Read the model definition and answer for the solid it produces. Units are mm, in the model's axes. Face numbers are marked on the shaded views. A direction names the side the tool comes from. Coordinates: 2 decimals unless noted, no trailing zeros. Loops run counter-clockwise (first coordinate to the right, second up) from the corner with the lowest first, then second, coordinate; pieces in that order, holes last.
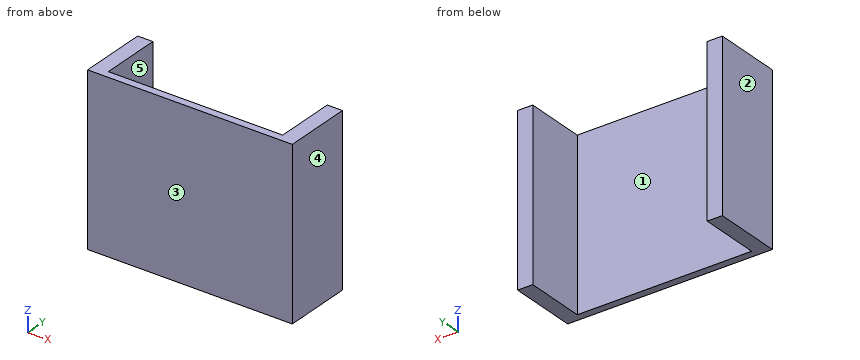
Autodesk Inventor part; units mm, degrees
ref_plane "YZ Plane" through (0, 0, 0) normal (1, 0, 0) x (0, 1, 0)
ref_plane "XZ Plane" through (0, 0, 0) normal (0, 1, 0) x (-1, 0, 0)
ref_plane "XY Plane" through (0, 0, 0) normal (0, 0, 1) x (1, 0, 0)
sketch "Sketch1" plane through (0, 0, 0) normal (0, 1, 0) x (-1, 0, 0)
  line L0 (86.4286, 125.7143) -> (-143.5714, 125.7143)
  line L1 (-143.5714, 125.7143) -> (-143.5714, -94.2857)
  line L2 (-143.5714, -94.2857) -> (86.4286, -94.2857)
  line L3 (86.4286, -94.2857) -> (86.4286, 125.7143)
  point P0 (0, 0)
  dimension "d0" = 220
  dimension "d1" = 230
extrude "Extrusion1" add sketch "Sketch1" along normal blind 10
sketch "Sketch5" plane through (-86.4286, 0, 125.7143) normal (0, 0, 1) x (1, 0, 0)
  line L0 (0, 0) -> (0, 10)
  line L1 (0, 0) -> (-20, 0)
  line L2 (-20, 0) -> (-20, 90)
  line L3 (-20, 90) -> (0, 90)
  line L4 (0, 90) -> (0, 0)
  line L5 (230, 0) -> (0, 0)
  line L6 (230, 0) -> (250, 0)
  line L7 (250, 0) -> (250, 90)
  line L8 (250, 90) -> (230, 90)
  line L9 (230, 90) -> (230, 0)
  point P0 (86.4286, 0)
  dimension "d22" = 90
  dimension "d23" = 20
  dimension "d24" = 20
extrude "Extrusion5" add sketch "Sketch5" against normal up to surface (220 mm away)
properties part number "Podkladka" material "Aluminum 6061"
Item 1: A cutting plane is placed at A-A on y = 23.5. Determine the outline of the cut face in (x, z).
Numbers:
outline: (-106.43, -94.29) - (-86.43, -94.29) - (-86.43, 125.71) - (-106.43, 125.71) - close; (143.57, -94.29) - (163.57, -94.29) - (163.57, 125.71) - (143.57, 125.71) - close
Item 2: A cutting plane is placed at B-B on z = 2.5. Determine the outline of the cut face in (x, y), then the cut area to 3 significant figures.
Numbers:
outline: (-106.43, 0) - (163.57, 0) - (163.57, 90) - (143.57, 90) - (143.57, 10) - (-86.43, 10) - (-86.43, 90) - (-106.43, 90) - close
area: 5,900 mm2
Item 3: Which of the six approach directions +Z, -Z, +X, -X, +Y, -Y give full straight-line access (tool end or side, diameter ignored) to the marked faces 1 and 2?
Numbers:
face 1: +Z, -Z, +Y
face 2: +Z, -Z, -X, +Y, -Y
Item 4: Given pin 1 (12 mm diameter, centred on x = 19.5, z = -72.5, fed in from +Y), flat-ended and moving along its own axis, determine where the tip first touches the part or whether it passes through.
Numbers:
pin 1: stops at y = 10
Item 5: Find the intervals of material crossed by line 1 along X through (y, z) = (82, -8); line 2 along Y through (x, z) = (57.5, 47), in increasing order.
Numbers:
line 1: x = -106.43 to -86.43, 143.57 to 163.57
line 2: y = 0 to 10
Item 6: Determine the mould class of the marked faces 3, 4 and 5 for opening direction X: released by +X, released by -X, zero draft, split by the parting line, or undercut.
Numbers:
face 3: zero draft
face 4: released by +X
face 5: undercut
Item 7: A cutting plane is placed at C-C on x = -8. Determine the outline of the cut face in (y, z), then the cut area to 3 significant figures.
Numbers:
outline: (0, -94.29) - (10, -94.29) - (10, 125.71) - (0, 125.71) - close
area: 2,200 mm2
